Model file for the job. Use its own axes, mm. A direction names the side the tool comes from. Coordinates: 2 decimals unless noted, no trailing zeros. Write each loop counter-clockwise with the first axis right and the second up, starting at its lowest first coordinate (ties: lowest second). Pieces come first, ordered by that corner, then holes. Notation, with made-up numbers: M 8.5,0.5 L 25.5,0.5 A24 ccw 25.5,22.5 Z; hole C 86.25,-31 d7. An arc over 180 degrees is marked long. One line per question, with ' | ' between items. Start each with the question number.
(1) Flat gauge pins, fed straight in: pin 1 Ø4 at (x, y) = (-18.5, -20.5) entering from -Z; pin 2 Ø1 at (y, z) = (18.5, 1.5) entering from -X; pin 3 Ø2 at (y, z) = (19, 2) entering from +X; pin 4 Ø9 at (x, y) = (19, 19) entering from +Z. Where does each tip first touch, or does it go through?
(2) Cut at C-C (z = 2.75). Write the cut outline in (x, y) (3 decimals).
(3) Cut at D-D (x = 20). Write the cut outline in (y, z).
(4) Tool access for faces 5 (the face through (-4.769, -21.477, 6.751)), 6 (the face through (16, 16, 2)), 7 (the face through (0.243, 24.723, 2.682)): list every direction of +Z, -Z, +X, -X, +Y, -Y with a clear straight run to the whole face (end or side of a thin tool).
(5) Cut at A-A (x = 0). Write the cut outline in (y, z) (3 decimals).
(6) Two-plate mould, pull along X, no slides. Class faces 1 (the face through (-17.18, -16.146, 3.696)), 2 (the face through (-12, 12, 0)), 3 (the face through (24.723, -0.246, 2.682)), 4 (the face through (12.804, -17.065, 0.986)): +X half, -X half, draft (parallel to the pull), parting line (faces both ways), or undercut.
(7) Wall check: probe 1 along X at (y, z) = (19, 3.75); probe 2 along X at (y, z) = (-20, 1.25); probe 3 along Z at (x, y) = (24.5, 21). Give the ranges that are in metal, low to high.
from build123d import *

# Parameters (mm, degrees)
SKETCH1_R           = 3.385
SKETCH1_R_2         = 16
BOSS_EXTRUDE1_DEPTH = 5.44
SKETCH2_R           = 6.5
CUT_EXTRUDE1_DEPTH  = 2
SKETCH3_R           = 22
BOSS_EXTRUDE2_DEPTH = 2.66
SKETCH4_R           = 13.635
CUT_EXTRUDE2_DEPTH  = 3.66


with BuildPart() as part:
    # Sketch1 → Boss-Extrude1 (new body)
    with BuildSketch(Plane.XY):
        with BuildLine():
            ThreePointArc((-17.15500238, -26.5786804), (-0.168836143, -24.722579211), (16.825003911, -26.507055409))
            ThreePointArc((16.825003911, -26.507055409), (24.281605458, -24.760439823), (26.649977107, -17.477419272))
            ThreePointArc((26.649977107, -17.477419272), (24.722401047, 0.0008954), (26.650274279, 17.479177295))
            ThreePointArc((26.650274279, 17.479177295), (24.514793015, 24.516072703), (17.477419272, 26.649977107))
            ThreePointArc((17.477419272, 26.649977107), (17.316247519, 26.614162818), (17.15500238, 26.5786804))
            ThreePointArc((17.15500238, 26.5786804), (0.000817995, 24.722401051), (-17.153414138, 26.578239095))
            ThreePointArc((-17.153414138, 26.578239095), (-17.316333175, 26.61408729), (-17.479177295, 26.650274279))
            ThreePointArc((-17.479177295, 26.650274279), (-24.516072703, 24.514793015), (-26.649977107, 17.477419272))
            ThreePointArc((-26.649977107, 17.477419272), (-24.722401047, -0.0008954), (-26.650274279, -17.479177295))
            ThreePointArc((-26.650274279, -17.479177295), (-24.514793015, -24.516072703), (-17.477419272, -26.649977107))
            ThreePointArc((-17.477419272, -26.649977107), (-17.316247519, -26.614162818), (-17.15500238, -26.5786804))
        make_face()
        with Locations((-18.999978097, -19.000021903)):
            Circle(SKETCH1_R, mode=Mode.SUBTRACT)
        with Locations((19.003521801, -19.017458637)):
            Circle(SKETCH1_R, mode=Mode.SUBTRACT)
        Circle(SKETCH1_R_2, mode=Mode.SUBTRACT)
        with Locations((-19.000021903, 18.999978097)):
            Circle(SKETCH1_R, mode=Mode.SUBTRACT)
        with Locations((18.999978097, 19.000021903)):
            Circle(SKETCH1_R, mode=Mode.SUBTRACT)
    extrude(amount=BOSS_EXTRUDE1_DEPTH)

    # Sketch2 → Cut-Extrude1 (cut)
    with BuildSketch(Plane(origin=(0, 0, 0), x_dir=(-1, 0, 0), z_dir=(0, 0, -1))):
        with Locations((19.000021903, 18.999978097)):
            Circle(SKETCH2_R)
        with Locations((-18.999978097, 19.000021903)):
            Circle(SKETCH2_R)
        with Locations((-19.003521801, -19.017458637)):
            Circle(SKETCH2_R)
        with Locations((18.999978097, -19.000021903)):
            Circle(SKETCH2_R)
    extrude(amount=-CUT_EXTRUDE1_DEPTH, mode=Mode.SUBTRACT)

    # Sketch3 → Boss-Extrude2 (add)
    with BuildSketch(Plane.XY.offset(5.44)):
        Circle(SKETCH3_R)
    extrude(amount=BOSS_EXTRUDE2_DEPTH)

    # Sketch4 → Cut-Extrude2 (cut, through all)
    with BuildSketch(Plane(origin=(0, 0, 5.44), x_dir=(-1, 0, 0), z_dir=(0, 0, -1))):
        Circle(SKETCH4_R)
    extrude(amount=-CUT_EXTRUDE2_DEPTH, mode=Mode.SUBTRACT)


solid = part.part
Filled in:
1) pin 1: z = 2 | pin 2: x = -26.8 | pin 3: x = 26.8 | pin 4: z = 5.44
2) outline: M -26.65,-17.479 A7.8 ccw -17.477,-26.65 A80.2 cw -17.155,-26.579 A80.2 cw 16.825,-26.507 A7.8 ccw 26.65,-17.477 A80.2 cw 26.65,17.479 A7.8 ccw 17.477,26.65 A80.2 cw 17.155,26.579 A80.2 cw -17.153,26.578 A80.2 cw -17.479,26.65 A7.8 ccw -26.65,17.477 A80.2 cw Z; hole C -19,-19 d6.77; hole C -19,19 d6.77; hole C 0,0 d32; hole C 19,19 d6.77; hole C 19.004,-19.017 d6.77
3) outline: M -26.75,0 L -25.44,0 L -25.44,2 L -22.25,2 L -22.25,5.44 L -26.75,5.44 Z; M -15.78,2 L -12.59,2 L -12.59,0 L 12.58,0 L 12.58,2 L 15.77,2 L 15.77,5.44 L 9.17,5.44 L 9.17,8.1 L -9.17,8.1 L -9.17,5.44 L -15.78,5.44 Z; M 22.23,2 L 25.42,2 L 25.42,0 L 26.74,0 L 26.74,5.44 L 22.23,5.44 Z
4) face 5: +Z | face 6: -Z | face 7: +Z, -Z, +Y
5) outline: M -24.722,0 L -16,0 L -16,5.44 L -13.635,5.44 L -13.635,8.1 L -22,8.1 L -22,5.44 L -24.722,5.44 Z; M 13.635,5.44 L 16,5.44 L 16,0 L 24.722,0 L 24.722,5.44 L 22,5.44 L 22,8.1 L 13.635,8.1 Z
6) face 1: undercut | face 2: draft | face 3: +X half | face 4: undercut
7) probe 1: -26.8 to -22.39, -15.62 to 15.61, 22.38 to 26.8 | probe 2: -26.74 to -25.42, -12.58 to 12.58, 25.43 to 26.74 | probe 3: 2 to 5.44
